```python
from build123d import *

# Parameters (mm, degrees)
BOSS_EXTRUDE1_DEPTH = 5.5
FILLET1_R           = 2.5


with BuildPart() as part:
    # Sketch1 → Boss-Extrude1 (new body)
    with BuildSketch(Plane(origin=(0, 0, 0), x_dir=(1, 0, 0), z_dir=(0, 1, 0))):
        Polygon((0, 0), (-10, 0), (-10, -15), (30, -15), (30, 0), (20, 0), (20, 8.5), (0, 8.5), align=None)
    extrude(amount=BOSS_EXTRUDE1_DEPTH)

    # Fillet1
    fillet1_edges = [part.edges().sort_by_distance(p)[0] for p in [
        (30, 2.75, 15),
        (-10, 2.75, 15),
    ]]
    fillet(fillet1_edges, radius=FILLET1_R)


solid = part.part
```
Read the model definition and answer for the solid it produces. Units are mm, in the model's axes. A direction names the side the tool comes from. Round coordinates to 2 decimals unless told otherwise and drop trailing zeros. Write each loop counter-clockwise with the first axis right and the second up, starting at its lowest first coordinate (ties: lowest second). Pieces come first, ordered by that corner, then holes. Notation, with made-up numbers: (76, 45.5) -> (83, 45.5) arc R27 cw to (83, 81.5) -> close; hole circle Ø9 at (50.5, 61.5). An arc over 180 degrees is marked (long way). Answer in a Markdown table with one row per item. Add a question column.
1) Consider line 1 (X direction, y = 3, z = -2); line 2 (Z direction, x = 25.5, y = 1.5); line 3 (Z direction, x = 28.5, y = 4). Determine where each line is inside the solid, lowest interval first.
2) Given P1, Ø3, axis at x = 22.5, y = 3.5, coming from the -Z side; P2, Ø3, axis at y = 1.5, z = -3.5, coming from the +X side, each flat-ended and moving along its own axis, determine where each tip first touches the part or whether it passes through.
3) Which of the six approach directions +Z, -Z, +X, -X, +Y, -Y give full straight-line access (tool end or side, diameter ignored) to faces 1 (the face through (25, 3, 0)), 2 (the face through (-10, 3, 6)), 3 (the face through (-5, 3, 0))?
4) Find section B-B, the plane z = -4.25. Determine the outline of the cut face in (x, y), and give its area (3 significant figures).
5) Find section A-A, the plane y = 4.7. Determine the outline of the cut face in (x, z).
6) Find section C-C, the plane x = 21. Determine the outline of the cut face in (y, z), and give its area (3 significant figures).
Findings below:
| question | item | result |
|---|---|---|
| 1 | line 1 | 0 to 20 |
| 1 | line 2 | 0 to 15 |
| 1 | line 3 | 0 to 14.79 |
| 2 | P1 | z = 0 |
| 2 | P2 | x = 20 |
| 3 | face 1 | -Z, +X, +Y, -Y |
| 3 | face 2 | +Z, -Z, -X, +Y, -Y |
| 3 | face 3 | -Z, -X, +Y, -Y |
| 4 | outline | (0, 0) -> (20, 0) -> (20, 5.5) -> (0, 5.5) -> close |
| 4 | area | 110 mm² |
| 5 | outline | (-10, 0) -> (0, 0) -> (0, -8.5) -> (20, -8.5) -> (20, 0) -> (30, 0) -> (30, 12.5) arc R2.5 ccw to (27.5, 15) -> (-7.5, 15) arc R2.5 ccw to (-10, 12.5) -> close |
| 6 | outline | (0, 0) -> (5.5, 0) -> (5.5, 15) -> (0, 15) -> close |
| 6 | area | 82.5 mm² |
